Could you check a few things on this model? Use its own coordinates, in mm. A direction names the side the tool comes from. Give positions to 0.01 mm unless a question says otherwise; leave off trailing zeros. Order: outer loops, then holes, each group sorted by start corner. A loop starts at its lowest first (then second) coordinate and runs counter-clockwise, first axis right, second up. Notation, with made-up numbers: (19.5, 54.25) - (58.5, 54.25) arc R18 ccw to (58.5, 62.25) - close; hole circle Ø1 at (45, 88). An arc over 180 degrees is marked (long way). Put each result on its own line as item: value.
from build123d import *

# Parameters (mm, degrees)
ESQUISSE1_R               = 3.5
ESQUISSE1_R_2             = 3
BOSS_EXTRU_1_DEPTH        = 3
BOSS_EXTRU_1_DEPTH_BACK   = 3
ESQUISSE1_R_3             = 9.5
ESQUISSE1_R_4             = 9
BOSS_EXTRU_1_2_DEPTH      = 3
BOSS_EXTRU_1_2_DEPTH_BACK = 3
ESQUISSE1_6_R             = 9
ESQUISSE1_6_R_2           = 3.5
BOSS_EXTRU_2_DEPTH        = 2.8
BOSS_EXTRU_2_DEPTH_BACK   = 2.8


with BuildPart() as part:
    # Esquisse1 → Boss.-Extru.1 (new body, two sides)
    with BuildSketch(Plane(origin=(0, 0, 0), x_dir=(1, 0, 0), z_dir=(0, 1, 0))) as boss_extru_1_sk:
        Circle(ESQUISSE1_R)
        Circle(ESQUISSE1_R_2, mode=Mode.SUBTRACT)
    extrude(amount=BOSS_EXTRU_1_DEPTH)
    extrude(boss_extru_1_sk.sketch, amount=-BOSS_EXTRU_1_DEPTH_BACK)



with BuildPart() as body_2:
    # Esquisse1 → Boss.-Extru.1 2 (new body, two sides)
    with BuildSketch(Plane(origin=(0, 0, 0), x_dir=(1, 0, 0), z_dir=(0, 1, 0))) as boss_extru_1_2_sk:
        Circle(ESQUISSE1_R_3)
        Circle(ESQUISSE1_R_4, mode=Mode.SUBTRACT)
    extrude(amount=BOSS_EXTRU_1_2_DEPTH)
    extrude(boss_extru_1_2_sk.sketch, amount=-BOSS_EXTRU_1_2_DEPTH_BACK)


with BuildPart() as part_1:
    add(part.part)

    add(body_2.part)  # Boss.-Extru.2 merges body 2
    # Esquisse1_6 → Boss.-Extru.2 (add, two sides)
    with BuildSketch(Plane(origin=(0, 0, 0), x_dir=(1, 0, 0), z_dir=(0, 1, 0))) as boss_extru_2_sk:
        Circle(ESQUISSE1_6_R)
        Circle(ESQUISSE1_6_R_2, mode=Mode.SUBTRACT)
    extrude(amount=BOSS_EXTRU_2_DEPTH)
    extrude(boss_extru_2_sk.sketch, amount=-BOSS_EXTRU_2_DEPTH_BACK)


solid = part_1.part
1) Suppose I cut it at C-C, the plane y = -1.1. List the corners of the cut face in (x, z) for me.
Filled in:
outline: circle Ø19 at (0, 0); hole circle Ø6 at (0, 0)
2) Suppose I cut it at A-A, the plane z = 0. List the corners of the cut face in (x, y) for me, and give its area (3 significant figures).
Filled in:
outline: (-9.5, -3) - (-9, -3) - (-9, -2.8) - (-3.5, -2.8) - (-3.5, -3) - (-3, -3) - (-3, 3) - (-3.5, 3) - (-3.5, 2.8) - (-9, 2.8) - (-9, 3) - (-9.5, 3) - close; (3, -3) - (3.5, -3) - (3.5, -2.8) - (9, -2.8) - (9, -3) - (9.5, -3) - (9.5, 3) - (9, 3) - (9, 2.8) - (3.5, 2.8) - (3.5, 3) - (3, 3) - close
area: 73.6 mm^2
3) Suppose I cut it at B-B, the plane x = 0. List the corners of the cut face in (y, z) for me, and give its area (3 significant figures).
Filled in:
outline: (-3, -9.5) - (3, -9.5) - (3, -9) - (2.8, -9) - (2.8, -3.5) - (3, -3.5) - (3, -3) - (-3, -3) - (-3, -3.5) - (-2.8, -3.5) - (-2.8, -9) - (-3, -9) - close; (-3, 3) - (3, 3) - (3, 3.5) - (2.8, 3.5) - (2.8, 9) - (3, 9) - (3, 9.5) - (-3, 9.5) - (-3, 9) - (-2.8, 9) - (-2.8, 3.5) - (-3, 3.5) - close
area: 73.6 mm^2
4) We'd pull the mould along X, two halves only. Please class faces 1 (the flat face through (3, -3, -1)), 2 (the cylindrical face through (4.38, 0.04, 8.43)), 3 (the flat face through (0, 2.8, 4)): pulls with the +X half, pulls with the -X half, needs draft (parallel to the pull), parting line crosses it, or undercut.
Filled in:
face 1: needs draft
face 2: parting line crosses it
face 3: undercut
5) Which directions (+Z, -Z, +X, -X, +Y, -Y) give clear straight access to the entire face, cutting with the end or side of a thin tool? Please do faces 4 (the flat face through (3, 3, -1)), 5 (the flat face through (0, -2.8, 4)).
Filled in:
face 4: +Z, -Z, +X, -X, +Y
face 5: -Y
6) I'm going to push flat-ended pins straight in: pin 1 (1 mm diameter, centred on x = 2, z = -6.5, fed in from -Y); pin 2 (3 mm diameter, centred on x = 7, y = -2, fed in from -Z); pin 3 (2 mm diameter, centred on x = 3.5, y = -2, fed in from -Z). Where does each tip first touch, or does it pass through?
Filled in:
pin 1: stops at y = -2.8
pin 2: stops at z = -7.75
pin 3: stops at z = -9.17
7) If I drill on line 1 (Z direction, x = 0, y = -2.85); line 2 (Y direction, x = 3.5, z = 4.5), over which ranges is the centre line in solid material (lowest first)? Write a range as [from, to].
Filled in:
line 1: z = [-9.5, -9], [-3.5, -3], [3, 3.5], [9, 9.5]
line 2: y = [-2.8, 2.8]
8) Suppose I cut it at D-D, the plane x = 5.75. List the corners of the cut face in (y, z) for me, and give its area (3 significant figures).
Filled in:
outline: (-3, -7.56) - (3, -7.56) - (3, -6.92) - (2.8, -6.92) - (2.8, 6.92) - (3, 6.92) - (3, 7.56) - (-3, 7.56) - (-3, 6.92) - (-2.8, 6.92) - (-2.8, -6.92) - (-3, -6.92) - close
area: 85.2 mm^2
